```python
from build123d import *

# Parameters (mm, degrees)
SKETCH1_R           = 4.5
SKETCH1_R_2         = 1
SKETCH1_R_3         = 1.5
BOSS_EXTRUDE1_DEPTH = 3


with BuildPart() as part:
    # Sketch1 → Boss-Extrude1 (new body)
    with BuildSketch(Plane.XY):
        with BuildLine():
            Line((0, 14), (70, 14))
            ThreePointArc((70, 14), (84, 0), (70, -14))
            Line((70, -14), (0, -14))
            ThreePointArc((0, -14), (-14, 0), (0, 14))
        make_face()
        Circle(SKETCH1_R, mode=Mode.SUBTRACT)
        with Locations((0, 8.5)):
            Circle(SKETCH1_R_2, mode=Mode.SUBTRACT)
        with Locations((8.5, 0)):
            Circle(SKETCH1_R_2, mode=Mode.SUBTRACT)
        with Locations((0, -8.5)):
            Circle(SKETCH1_R_2, mode=Mode.SUBTRACT)
        with Locations((-8.5, 0)):
            Circle(SKETCH1_R_2, mode=Mode.SUBTRACT)
        with Locations((70, 0)):
            Circle(SKETCH1_R, mode=Mode.SUBTRACT)
        with Locations((70, 8.5)):
            Circle(SKETCH1_R_2, mode=Mode.SUBTRACT)
        with Locations((78.5, 0)):
            Circle(SKETCH1_R_2, mode=Mode.SUBTRACT)
        with Locations((70, -8.5)):
            Circle(SKETCH1_R_2, mode=Mode.SUBTRACT)
        with Locations((61.5, 0)):
            Circle(SKETCH1_R_2, mode=Mode.SUBTRACT)
        with Locations((25, 0)):
            Circle(SKETCH1_R_3, mode=Mode.SUBTRACT)
        with Locations((35, 0)):
            Circle(SKETCH1_R_3, mode=Mode.SUBTRACT)
        with Locations((45, 0)):
            Circle(SKETCH1_R_3, mode=Mode.SUBTRACT)
    extrude(amount=BOSS_EXTRUDE1_DEPTH)


solid = part.part
```
Model file for the job. Use its own axes, mm. Round coordinates to 2 decimals unless told otherwise and drop trailing zeros. Write each loop counter-clockwise with the first axis right and the second up, starting at its lowest first coordinate (ties: lowest second). Pieces come first, ordered by that corner, then holes. Notation, with made-up numbers: M -26,-4 L -14,-4 A33 ccw -14,30 Z; hole C -35,-20 d8. An arc over 180 degrees is marked long. Put each result on its own line as item: value.
Item 1: Cut at A-A (x = 25). List the corners of the cut face in (y, z).
Responses:
outline: M -14,0 L -1.5,0 L -1.5,3 L -14,3 Z; M 1.5,0 L 14,0 L 14,3 L 1.5,3 Z
Item 2: Cut at D-D (x = 61.5). List the corners of the cut face in (y, z).
Responses:
outline: M -14,0 L -1,0 L -1,3 L -14,3 Z; M 1,0 L 14,0 L 14,3 L 1,3 Z
Item 3: Probe L1, parallel to Y at x = 25, z = 2.1; L2, parallel to Y at x = 72, z = 2.8; L3, parallel to X at y = -3, z = 2.7. List the from-to ranges inside material, lowest first. Write a range as from..to.
Responses:
L1: -14..-1.5, 1.5..14
L2: -13.86..-4.03, 4.03..13.86
L3: -13.67..-3.35, 3.35..66.65, 73.35..83.67
Item 4: Mould opens along X. For faces 1 (the flat face through (36, 3, 3)), 2 (the cylindrical face through (60.5, 0, 1.5)), 3 (the cylindrical face through (-9.3, -0.6, 1.5)), 4 (the cylindrical face through (84, 0, 1)) say: +X half, -X half, draft (parallel to the pull), parting line (faces both ways), or undercut.
Responses:
face 1: draft
face 2: undercut
face 3: undercut
face 4: +X half
Item 5: Flat gauge pin, fed straight in: P1, Ø8, axis at x = 0, y = 0, coming from the -Z side. Where does the tip first touch, or does it go through?
Responses:
P1: through
Item 6: Cut at C-C (z = 1.15). State how many separate pieces and enclosed holes the cut face has, and give its area (3 significant figures).
Responses:
separate pieces: 1
enclosed holes: 13
area: 2,400 mm²
Item 7: Cut at B-B (y = 8.5). List the corners of the cut face in (x, z).
Responses:
outline: M -11.12,0 L -1,0 L -1,3 L -11.12,3 Z; M 1,0 L 69,0 L 69,3 L 1,3 Z; M 71,0 L 81.12,0 L 81.12,3 L 71,3 Z
